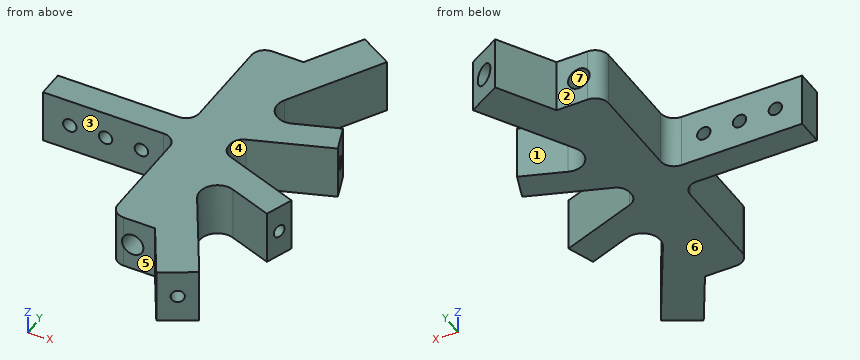
```python
from build123d import *

# Parameters (mm, degrees)
EXTRUDE_1_DEPTH      = 6
FILLET_4_R           = 1.5
FILLET_5_R           = 2
SKETCH_7_R           = 1.2
CUT_EXTRUDE_6_DEPTH  = 10
SKETCH_8_R           = 0.7
CUT_EXTRUDE_7_DEPTH  = 10
SKETCH_9_R           = 0.7
CUT_EXTRUDE_8_DEPTH  = 10
SKETCH_10_R          = 0.7
CUT_EXTRUDE_9_DEPTH  = 10
CUT_EXTRUDE_10_REACH = 42.531
SKETCH_11_R          = 1.2
FILLET_6_R           = 1.5
CUT_EXTRUDE_11_REACH = 31.177
SKETCH_12_R          = 0.75


with BuildPart() as part:
    # 草圖1 → 填料-伸長1 (new body)
    with BuildSketch(Plane.XY):
        Polygon((-2.5, 15), (2.5, 15), (6, 21.062177826), (9.637306696, 18.962177826), (2.5, 6.6), (2.5, 4.605368872), (10.957233587, 7.683550162), (12.051698046, 4.676533775), (2.5, 1.2), (2.5, -1.2), (12.051698046, -4.676533775), (10.957233587, -7.683550162), (2.5, -4.605368872), (2.5, -6.6), (9.637306696, -18.962177826), (6, -21.062177826), (2.5, -15), (-2.5, -15), (-2.5, -1.5), (-17.5, -1.5), (-17.5, 1.5), (-2.5, 1.5), align=None)
    extrude(amount=EXTRUDE_1_DEPTH)

    # 圓角4
    # the kernel refuses this fillet: 1.5 mm, written as the material it adds along each edge
    with BuildSketch(Plane(origin=(-2.5, -1.5, 0), x_dir=(0, -1, 0), z_dir=(0, 0, 1)), Plane(origin=(-2.5, 1.5, 0), x_dir=(-1, 0, 0), z_dir=(0, 0, 1))) as fillet_4_piece_1:
        with BuildLine():
            CenterArc((FILLET_4_R, -FILLET_4_R), FILLET_4_R, 90, 90)
            Line((0, -FILLET_4_R), (-FILLET_4_R * 0.02, -FILLET_4_R))
            Line((-FILLET_4_R * 0.02, -FILLET_4_R), (-FILLET_4_R * 0.02, FILLET_4_R * 0.02))
            Line((-FILLET_4_R * 0.02, FILLET_4_R * 0.02), (FILLET_4_R, FILLET_4_R * 0.02))
            Line((FILLET_4_R, FILLET_4_R * 0.02), (FILLET_4_R, 0))
        make_face()
    extrude(amount=6)
    with BuildSketch(Plane(origin=(2.5, 4.605368872, 0), x_dir=(0, 1, 0), z_dir=(0, 0, 1))) as fillet_4_piece_2:
        with BuildLine():
            CenterArc((2.139664035, -1.492972021), FILLET_4_R, 95.548517206, 104.451482794)
            Line((0.730125104, -2.006002236), (0.701934325, -2.01626284))
            Line((0.701934325, -2.01626284), (-0.028190779, -0.010260604))
            Line((-0.028190779, -0.010260604), (0, 0.03))
            ThreePointArc((0, 0.03), (0.997315564, 0.03), (1.99173047, 0.02985944))
            Line((1.99173047, 0.02985944), (1.994631128, 0))
        make_face()
    extrude(amount=6)
    with BuildSketch(Plane(origin=(2.5, 1.2, 0), x_dir=(0.9396926207859073, 0.34202014332567154, 0), z_dir=(0, 0, 1)), Plane(origin=(2.5, -1.2, 0), x_dir=(0, 1, 0), z_dir=(0, 0, 1))) as fillet_4_piece_3:
        with BuildLine():
            CenterArc((FILLET_4_R * 0.70020753821, -FILLET_4_R), FILLET_4_R, 90, 70)
            Line((-FILLET_4_R * 0.239485082576, -FILLET_4_R * 0.657979856674), (-FILLET_4_R * 0.258278934992, -FILLET_4_R * 0.651139453808))
            Line((-FILLET_4_R * 0.258278934992, -FILLET_4_R * 0.651139453808), (-FILLET_4_R * 0.0140041507642, FILLET_4_R * 0.02))
            Line((-FILLET_4_R * 0.0140041507642, FILLET_4_R * 0.02), (FILLET_4_R * 0.70020753821, FILLET_4_R * 0.02))
            Line((FILLET_4_R * 0.70020753821, FILLET_4_R * 0.02), (FILLET_4_R * 0.70020753821, 0))
        make_face()
    extrude(amount=6)
    with BuildSketch(Plane(origin=(2.5, -4.605368872, 0), x_dir=(0.9396926207859109, -0.34202014332566216, 0), z_dir=(0, 0, 1))) as fillet_4_piece_4:
        with BuildLine():
            CenterArc((2.134742991, -1.5), FILLET_4_R, 90, 104.451482794)
            Line((0.682204024, -1.874340152), (0.653153245, -1.881826955))
            ThreePointArc((0.653153245, -1.881826955), (0.312911234, -0.94743068), (-0.028190779, -0.010260604))
            Line((-0.028190779, -0.010260604), (0, 0.03))
            Line((0, 0.03), (2.134742991, 0.03))
            Line((2.134742991, 0.03), (2.134742991, 0))
        make_face()
    extrude(amount=6)

    # 圓角5
    fillet_5_edges = [part.edges().sort_by_distance(p)[0] for p in [
        (2.5, -6.6, 3),
        (2.5, 6.6, 3),
    ]]
    fillet(fillet_5_edges, radius=FILLET_5_R)

    # 草圖7 → 除料-伸長6 (cut)
    with BuildSketch(Plane(origin=(10.620190528, 18.394709581, 0), x_dir=(0.8660254037844364, -0.5000000000000041, 0), z_dir=(0.5000000000000041, 0.8660254037844364, 0))):
        with Locations(Location((-3.234936491, -3, 0), (0, 0, 180))):
            Circle(SKETCH_7_R)
    extrude(amount=-CUT_EXTRUDE_6_DEPTH, mode=Mode.SUBTRACT)

    # 草圖8 → 除料-伸長7 (cut)
    with BuildSketch(Plane(origin=(10.620190528, -18.394709581, 0), x_dir=(0.8660254037844356, 0.5000000000000054, 0), z_dir=(0.5000000000000054, -0.8660254037844356, 0))):
        with Locations((-3.234936491, 3)):
            Circle(SKETCH_8_R)
    extrude(amount=-CUT_EXTRUDE_7_DEPTH, mode=Mode.SUBTRACT)

    # 草圖9 → 除料-伸長8 (cut)
    with BuildSketch(Plane(origin=(12.144926165, -4.420391622, 0), x_dir=(0, 0, -1), z_dir=(0.9396926207859106, -0.3420201433256625, 0))):
        with Locations(Location((-3, -1.872580787, 0), (0, 0, 90))):
            Circle(SKETCH_9_R)
    extrude(amount=-CUT_EXTRUDE_8_DEPTH, mode=Mode.SUBTRACT)

    # 草圖10 → 除料-伸長9 (cut)
    with BuildSketch(Plane(origin=(12.144926165, 4.420391622, 0), x_dir=(0, 0, -1), z_dir=(0.9396926207859082, 0.3420201433256692, 0))):
        with Locations(Location((-3, 1.872580787, 0), (0, 0, 90))):
            Circle(SKETCH_10_R)
    extrude(amount=-CUT_EXTRUDE_9_DEPTH, mode=Mode.SUBTRACT)

    # 草圖11 → 除料-伸長10 (cut, up to next)
    with BuildSketch(Plane.XZ.offset(15), mode=Mode.PRIVATE) as cut_extrude_10_sk1:
        with Locations(Location((0, 3, 0), (0, 0, 270))):
            Circle(SKETCH_11_R)
    cut_extrude_10_tool1 = extrude(cut_extrude_10_sk1.sketch, amount=-CUT_EXTRUDE_10_REACH, mode=Mode.PRIVATE) & part.part
    add(cut_extrude_10_tool1.solids().sort_by_distance((0, -15, 3))[0], mode=Mode.SUBTRACT)

    # 圓角6
    # the kernel refuses this fillet: 1.5 mm, written as the material it takes off along each edge
    with BuildSketch(Plane(origin=(-2.5, -15, -3.75), x_dir=(1, 0, 0), z_dir=(0, 0, 1)), Plane(origin=(-2.5, 15, -3.75), x_dir=(0, -1, 0), z_dir=(0, 0, 1))) as fillet_6_piece_1:
        with BuildLine():
            CenterArc((FILLET_6_R, FILLET_6_R), FILLET_6_R, 180, 90)
            Line((0, FILLET_6_R), (0, 0))
            Line((0, 0), (FILLET_6_R, 0))
        make_face()
    extrude(amount=13.5, mode=Mode.SUBTRACT)

    # 草圖12 → 除料-伸長11 (cut, up to next)
    with BuildSketch(Plane.XZ.offset(1.5), mode=Mode.PRIVATE) as cut_extrude_11_sk1:
        with Locations((-6.5, 3)):
            Circle(SKETCH_12_R)
    cut_extrude_11_tool1 = extrude(cut_extrude_11_sk1.sketch, amount=-CUT_EXTRUDE_11_REACH, mode=Mode.PRIVATE) & part.part
    # 草圖12 → 除料-伸長11 (cut, up to next)
    with BuildSketch(Plane.XZ.offset(1.5), mode=Mode.PRIVATE) as cut_extrude_11_sk2:
        with Locations((-10.5, 3)):
            Circle(SKETCH_12_R)
    cut_extrude_11_tool2 = extrude(cut_extrude_11_sk2.sketch, amount=-CUT_EXTRUDE_11_REACH, mode=Mode.PRIVATE) & part.part
    # 草圖12 → 除料-伸長11 (cut, up to next)
    with BuildSketch(Plane.XZ.offset(1.5), mode=Mode.PRIVATE) as cut_extrude_11_sk3:
        with Locations((-14.5, 3)):
            Circle(SKETCH_12_R)
    cut_extrude_11_tool3 = extrude(cut_extrude_11_sk3.sketch, amount=-CUT_EXTRUDE_11_REACH, mode=Mode.PRIVATE) & part.part
    add(cut_extrude_11_tool1.solids().sort_by_distance((-6.5, -1.5, 3))[0], mode=Mode.SUBTRACT)
    add(cut_extrude_11_tool2.solids().sort_by_distance((-10.5, -1.5, 3))[0], mode=Mode.SUBTRACT)
    add(cut_extrude_11_tool3.solids().sort_by_distance((-14.5, -1.5, 3))[0], mode=Mode.SUBTRACT)


solid = part.part
```
Could you check a few things on this model? Use its own coordinates, in mm. Face numbers are marked on the shaded views. A direction names the side the tool comes from. Round coordinates to 2 decimals unless told otherwise and drop trailing zeros. Loops run counter-clockwise (first coordinate to the right, second up) from the corner with the lowest first, then second, coordinate; pieces in that order, holes last. Notation, with made-up numbers: (78, -2.75) - (104, -2.75) arc R13 cw to (104, 11.25) - close; hole circle Ø8 at (-9.5, -40). An arc over 180 degrees is marked (long way). Use CSV: the item, a comma, the result in double quotes.
Item 1: Will these pins go through, and if not, where does the flat tip stop? pin 1 (1.5 mm diameter, centred on x = -5.5, z = 3, fed in from -Y); pin 2 (1.8 mm diameter, centred on y = -9.5, z = 3, fed in from -X); pin 3 (1.9 mm diameter, centred on x = 0, z = 3, fed in from +Y); pin 4 (1.1 mm diameter, centred on x = 0.5, z = 4, fed in from +Y).
Here are the results:
pin 1,"stops at y = -1.5"
pin 2,"stops at x = -2.5"
pin 3,"passes through"
pin 4,"stops at y = 15"
Item 2: If we section it at B-B on x = -8: List the corners of the cut face in (y, z) for me.
Here are the results:
outline,"(-1.5, 0) - (1.5, 0) - (1.5, 6) - (-1.5, 6) - close"
Item 3: For the marked faces 1, 2, 3 and 4, which set-ups out of +Z, -Z, +X, -X, +Y, -Y let a thin tool reach every point of the face, with its end or its side?
Here are the results:
face 1,"+Z, -Z"
face 2,"+Z, -Z, -X, +Y"
face 3,"+Z, -Z, -X, -Y"
face 4,"+Z, -Z, +X"
Item 4: I need wall thicknesses on L1, parallel to Z at x = -6.5, y = -0.4; L2, parallel to Y at x = 9.5, z = 3.25; L3, parallel to Y at x = -8, z = 4.25. Which ranges of each line are inside material? Lowest first, please. Write a range as [from, to].
Here are the results:
L1,"z = [0, 2.25], [3.75, 6]"
L2,"y = [-19.04, -18.72], [-7.15, -6.15], [-4.75, -3.75], [3.75, 4.75], [6.15, 7.15], [18.72, 19.04]"
L3,"y = [-1.5, 1.5]"
Item 5: If we section it at A-A on x = -14.5: List the corners of the cut face in (y, z) for me.
Here are the results:
outline,"(-1.5, 0) - (1.5, 0) - (1.5, 2.25) - (-1.5, 2.25) - close; (-1.5, 3.75) - (1.5, 3.75) - (1.5, 6) - (-1.5, 6) - close"
Item 6: If we mould it in two halves opening along Z, with no side actions, what happens to the marked faces 5, 6 and 7? For each: pulls with the +Z half, pulls with the -Z half, needs draft (parallel to the pull), parting line crosses it, or undercut.
Here are the results:
face 5,"needs draft"
face 6,"pulls with the -Z half"
face 7,"undercut"
